```python
from build123d import *

# Parameters (mm, degrees)
SKETCH1_W                      = 12.7
SKETCH1_H                      = 12.7
BOSS_EXTRUDE1_DEPTH            = 4.1275
SKETCH2_R                      = 2.9718
CUT_EXTRUDE1_DEPTH             = 15.786776398
SKETCH3_R                      = 3.96875
BOSS_EXTRUDE2_DEPTH            = 12.7
SKETCH4_OUTSIDE_W              = 20.22
SKETCH4_OUTSIDE_H              = 20.22
SKETCH4_OUTSIDE_R              = 3.2385
CUT_EXTRUDE2_DEPTH             = 3.937
BOSS_EXTRUDE3_START            = 3.048
SKETCH5_R                      = 3.96875
BOSS_EXTRUDE3_DEPTH            = 3.048
CHAMFER1_SIZE                  = 1.75
CHAMFER1_SIZE2                 = 3.031088913
SKETCH6_R                      = 0.175
CUT_EXTRUDE3_DEPTH             = 26.627895134
F_3_5_3_5_DIAMETER_HOLE1_D     = 3.5
F_3_5_3_5_DIAMETER_HOLE1_DEPTH = 21
F_3_5_3_5_DIAMETER_HOLE1_TIP   = 1.051506083
SKETCH11_R                     = 1.143
CUT_EXTRUDE4_DEPTH             = 4


with BuildPart() as part:
    # Sketch1 → Boss-Extrude1 (new, symmetric)
    with BuildSketch(Plane.XY):
        Rectangle(SKETCH1_W, SKETCH1_H)
    extrude(amount=BOSS_EXTRUDE1_DEPTH, both=True)

    # Sketch2 → Cut-Extrude1 (cut, through all)
    with BuildSketch(Plane.XZ.offset(6.35)):
        with Locations(Location((2.8448, 0, 0), (0, 0, 270))):
            Circle(SKETCH2_R)
    extrude(amount=-CUT_EXTRUDE1_DEPTH, mode=Mode.SUBTRACT)

    # Sketch3 → Boss-Extrude2 (add)
    with BuildSketch(Plane.XY.offset(4.1275)):
        with Locations(Location((-2.38125, 0, 0), (0, 0, 180))):
            Circle(SKETCH3_R)
    extrude(amount=BOSS_EXTRUDE2_DEPTH)

    # Sketch4 outside → Cut-Extrude2 (cut)
    with BuildSketch(Plane.XY.offset(16.8275)):
        Rectangle(SKETCH4_OUTSIDE_W, SKETCH4_OUTSIDE_H)
        with Locations((-2.38125, 0)):
            Circle(SKETCH4_OUTSIDE_R, mode=Mode.SUBTRACT)
    extrude(amount=-CUT_EXTRUDE2_DEPTH, mode=Mode.SUBTRACT)

    # Sketch5 → Boss-Extrude3 (add)
    with BuildSketch(Plane(origin=(0, 0, -4.1275), x_dir=(-1, 0, 0), z_dir=(0, 0, -1)).offset(BOSS_EXTRUDE3_START)):
        with Locations((2.38125, 0)):
            Circle(SKETCH5_R)
    extrude(amount=-BOSS_EXTRUDE3_DEPTH)

    # Chamfer1
    chamfer1_edges = [part.edges().sort_by_distance(p)[0] for p in [
        (1.5875, 0, -7.1755),
    ]]
    chamfer1_side = [part.faces().sort_by_distance(p)[0] for p in [
        (1.5875, 0, -5.6515),
    ]]
    chamfer(chamfer1_edges, length=CHAMFER1_SIZE, length2=CHAMFER1_SIZE2, reference=chamfer1_side[0])

    # Sketch6 → Cut-Extrude3 (cut, through all)
    with BuildSketch(Plane(origin=(0, 0, -7.1755), x_dir=(-1, 0, 0), z_dir=(0, 0, -1))):
        with Locations((2.38125, 0)):
            Circle(SKETCH6_R)
    extrude(amount=-CUT_EXTRUDE3_DEPTH, mode=Mode.SUBTRACT)

    # Ø3.5 (3.5) Diameter Hole1
    with Locations(Plane.XY.offset(16.8275)):
        with Locations((-2.38125, 0)):
            Hole(F_3_5_3_5_DIAMETER_HOLE1_D / 2, depth=F_3_5_3_5_DIAMETER_HOLE1_DEPTH)
            with Locations((0, 0, -(F_3_5_3_5_DIAMETER_HOLE1_DEPTH + F_3_5_3_5_DIAMETER_HOLE1_TIP / 2))):  # 118° drill point
                Cone(0, F_3_5_3_5_DIAMETER_HOLE1_D / 2, F_3_5_3_5_DIAMETER_HOLE1_TIP, mode=Mode.SUBTRACT)

    # Sketch11 → Cut-Extrude4 (cut)
    with BuildSketch(Plane.ZY.offset(6.35)):
        with Locations((-0.8725, 4.35)):
            Circle(SKETCH11_R)
    extrude(amount=-CUT_EXTRUDE4_DEPTH, mode=Mode.SUBTRACT)


solid = part.part
```
For this review, take the finished solid that the model builds, in its own axes (mm). A direction names the side the tool comes from. Round coordinates to 2 decimals unless told otherwise and drop trailing zeros. Write each loop counter-clockwise with the first axis right and the second up, starting at its lowest first coordinate (ties: lowest second). Pieces come first, ordered by that corner, then holes. Notation, with made-up numbers: (4.5, 21.25) - (26.5, 21.25) arc R12 cw to (26.5, 29.25) - close; hole circle Ø1 at (9.25, 8.5). An arc over 180 degrees is marked (long way). Answer as a JSON object with one key per item and string values.
1. We need section D-D on z = 12. Give the boundary of the cut face in (x, y).
Response values:
{"outline": "circle Ø7.94 at (-2.38, 0); hole circle Ø3.5 at (-2.38, 0)"}
2. To check wall thickness, follow line 1 along X through (y, z) = (0, 0); line 2 along Y through (x, z) = (-2.5, 13.25); line 3 along X through (y, z) = (-1.5, 0). State the ranges of each line that lie inside material, in increasing order.
Response values:
{"line 1": "x = -6.35 to -4.13, -0.63 to -0.13, 5.82 to 6.35", "line 2": "y = -3.24 to -1.75, 1.75 to 3.24", "line 3": "x = -6.35 to -3.28, -1.48 to -0.13, 5.82 to 6.35"}
3. We need section A-A on z = 0. Give the boundary of the cut face in (x, y), then the cut area to 3 significant figures.
Response values:
{"outline": "(-6.35, -6.35) - (-0.13, -6.35) - (-0.13, 6.35) - (-6.35, 6.35) - (-6.35, 5.09) - (-2.35, 5.09) - (-2.35, 3.61) - (-6.35, 3.61) - close; (5.82, -6.35) - (6.35, -6.35) - (6.35, 6.35) - (5.82, 6.35) - close; hole circle Ø3.5 at (-2.38, 0)", "area": "70.3 mm2"}
4. We need section C-C on y = 4.35. Give the boundary of the cut face in (x, z).
Response values:
{"outline": "(-6.35, -4.13) - (6.35, -4.13) - (6.35, 4.13) - (-6.35, 4.13) - (-6.35, 0.27) - (-2.35, 0.27) - (-2.35, -2.02) - (-6.35, -2.02) - close; hole circle Ø5.94 at (2.84, 0)"}
5. We need section B-B on x = 4. Give the boundary of the cut face in (y, z).
Response values:
{"outline": "(-6.35, -4.13) - (6.35, -4.13) - (6.35, -2.74) - (-6.35, -2.74) - close; (-6.35, 2.74) - (6.35, 2.74) - (6.35, 4.13) - (-6.35, 4.13) - close"}
6. For pin 1 Ø3 at (x, y) = (-0.5, -5) entering from -Z; pin 2 Ø2 at (y, z) = (2.5, -4.5) entering from -X; pin 3 Ø2 at (x, z) = (-4, 12) entering from -Y; pin 4 Ø1.1 at (y, z) = (4, -1) entering from -X, all flat-tipped, find the tip position at first contact; note any pin that passes through.
Response values:
{"pin 1": "stops at z = -5.5", "pin 2": "stops at x = -6.35", "pin 3": "stops at y = -3.92", "pin 4": "stops at x = -2.35"}
7. Draft analysis for pull direction X (two halves, no side actions). For faces 5 (the face through (-2, 6.35, 0)), 6 (the face through (5.35, -0.09, -1.6)), 7 (the face through (0.77, 2.41, 8.45)), state which applies: +X half, -X half, draft (parallel to the pull), parting line (faces both ways), or undercut.
Response values:
{"face 5": "draft", "face 6": "undercut", "face 7": "parting line"}
8. Tool access review of faces 1 (the face through (-4.378, 3.336, -0.345)), 2 (the face through (1.584, 0.174, -4.786)), 3 (the face through (-4.05, 0.53, 6.18)), 4 (the face through (-6.35, 0, 0)): name each direction out of +Z, -Z, +X, -X, +Y, -Y from which nothing blocks a thin tool from reaching the whole face with its end or side.
Response values:
{"face 1": "-X", "face 2": "-Z", "face 3": "+Z", "face 4": "+Z, -Z, -X, +Y, -Y"}
